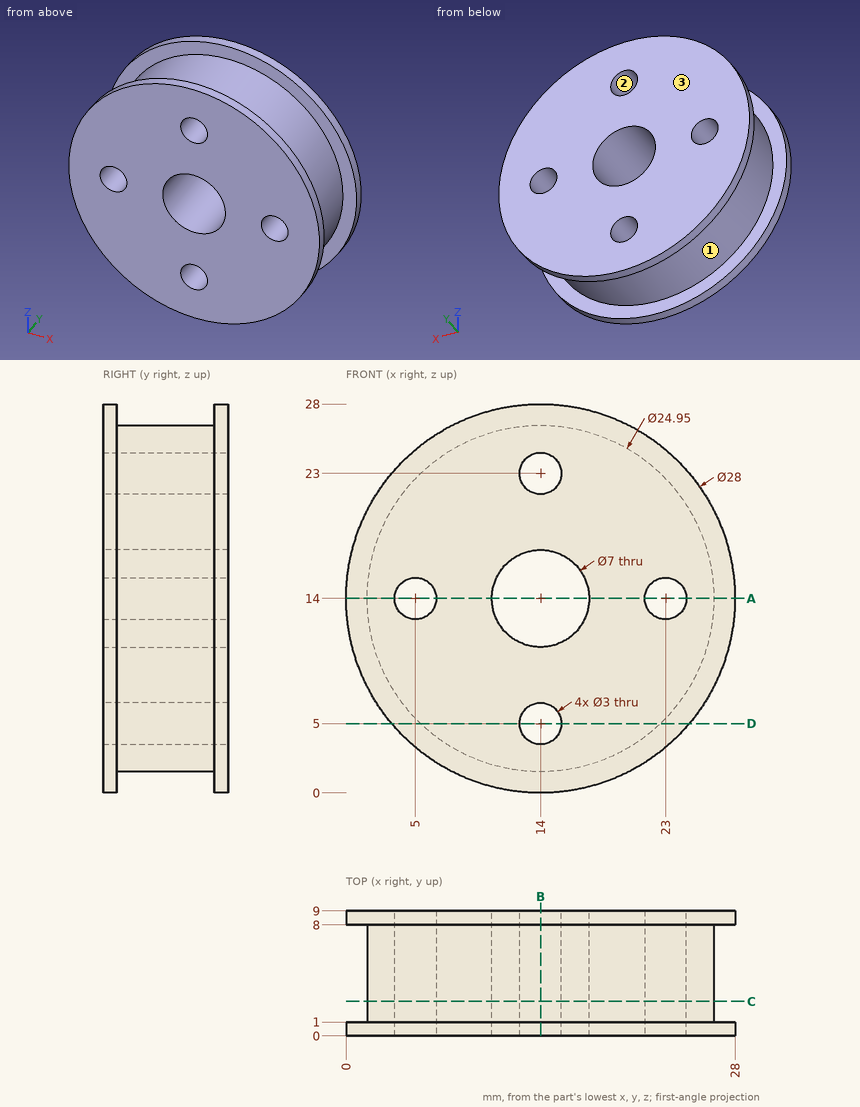
Answer from the drawing. Dimensions are ordinates in mm from the lowest x, y and z of the part. Round coordinates to 2 decimals unless told otherwise and drop trailing zeros. Loops run counter-clockwise (first coordinate to the right, second up) from the corner with the lowest first, then second, coordinate; pieces in that order, holes last.
1) Consider line 1 (X direction, y = 3, z = 14.25); line 2 (Y direction, x = 5.75, z = 3.25); line 3 (Z direction, x = 22.75, y = 4.25). Determine where each line is inside the solid, lowest interval first.
Outcome:
line 1: x = 1.53 to 3.52, 6.48 to 10.51, 17.49 to 21.52, 24.48 to 26.47
line 2: y = 0 to 1, 8 to 9
line 3: z = 5.11 to 12.52, 15.48 to 22.89
2) A cutting plane is placed at C-C on y = 2.5. Determine the outline of the cut face in (x, z) (3 decimals).
Outcome:
outline: circle Ø24.95 at (14, 14); hole circle Ø3 at (5, 14); hole circle Ø7 at (14, 14); hole circle Ø3 at (14, 5); hole circle Ø3 at (14, 23); hole circle Ø3 at (23, 14)
3) Given P1, Ø1, axis at y = 6.5, z = 18.5, coming from the -X side; P2, Ø2, axis at x = 22.5, y = 2.5, coming from the +Z side; P3, Ø1, axis at y = 6, z = 20, coming from the -X side, each flat-ended and moving along its own axis, determine where each tip first touches the part or whether it passes through.
Outcome:
P1: stops at x = 2.18
P2: stops at z = 23.97
P3: stops at x = 2.8
4) A cutting plane is placed at D-D on z = 5. Determine the outline of the cut face in (x, y), plus the area to 3 significant figures.
Outcome:
outline: (3.28, 0) - (12.5, 0) - (12.5, 9) - (3.28, 9) - (3.28, 8) - (5.36, 8) - (5.36, 1) - (3.28, 1) - close; (15.5, 0) - (24.72, 0) - (24.72, 1) - (22.64, 1) - (22.64, 8) - (24.72, 8) - (24.72, 9) - (15.5, 9) - close
area: 137 mm2
5) A cutting plane is placed at B-B on x = 14. Determine the outline of the cut face in (y, z) (3 decimals), plus the area to 3 significant figures.
Outcome:
outline: (0, 0) - (1, 0) - (1, 1.525) - (8, 1.525) - (8, 0) - (9, 0) - (9, 3.5) - (0, 3.5) - close; (0, 6.5) - (9, 6.5) - (9, 10.5) - (0, 10.5) - close; (0, 17.5) - (9, 17.5) - (9, 21.5) - (0, 21.5) - close; (0, 24.5) - (9, 24.5) - (9, 28) - (8, 28) - (8, 26.475) - (1, 26.475) - (1, 28) - (0, 28) - close
area: 114 mm2
6) A cutting plane is placed at A-A on z = 14. Determine the outline of the cut face in (x, y) (3 decimals), plus the area to 3 significant figures.
Outcome:
outline: (0, 0) - (3.5, 0) - (3.5, 9) - (0, 9) - (0, 8) - (1.525, 8) - (1.525, 1) - (0, 1) - close; (6.5, 0) - (10.5, 0) - (10.5, 9) - (6.5, 9) - close; (17.5, 0) - (21.5, 0) - (21.5, 9) - (17.5, 9) - close; (24.5, 0) - (28, 0) - (28, 1) - (26.475, 1) - (26.475, 8) - (28, 8) - (28, 9) - (24.5, 9) - close
area: 114 mm2
7) For a pull along Z with two mould halves and no side action, classify the marked faces 1, 2 and 3 as released by +Z, released by -Z, zero draft, split by the parting line, or undercut.
Outcome:
face 1: split by the parting line
face 2: undercut
face 3: zero draft
